Design review of the part built by this model. Coordinates are the model's own, in mm. Face numbers are marked on the shaded views. Give positions to 0.01 mm unless a question says otherwise; leave off trailing zeros. Write each loop counter-clockwise with the first axis right and the second up, starting at its lowest first coordinate (ties: lowest second). Pieces come first, ordered by that corner, then holes. Notation, with made-up numbers: M 17,54 L 34,54 A17 ccw 34,68 Z; hole C 20,-36.5 d11. An arc over 180 degrees is marked long. Use a Markdown table: item, result. Add a question column.
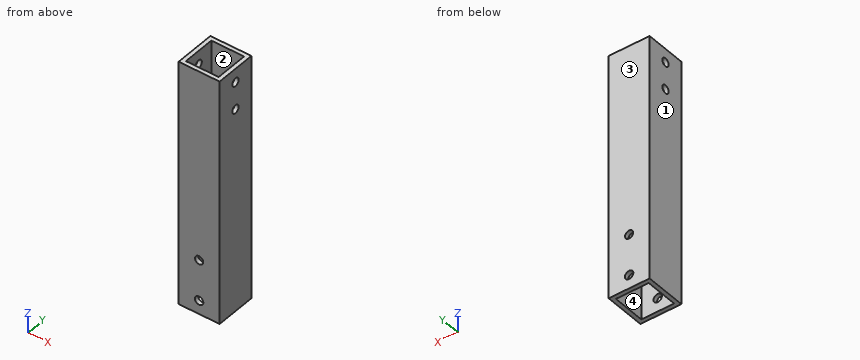
```python
from build123d import *

# Parameters (mm, degrees)
ESQUISSE1_W             = 15
ESQUISSE1_H             = 15
EXTRUSION1_DEPTH        = 90
ESQUISSE2_W             = 12
ESQUISSE2_H             = 12
EXTRUSION2_DEPTH        = 91.622844802
ESQUISSE3_R             = 1.5
ENL_V_MAT_EXTRU_1_DEPTH = 92.549167118
ESQUISSE4_R             = 1.5
ESQUISSE4_R_2           = 1.538778498
ENL_V_MAT_EXTRU_2_DEPTH = 92.549167118


with BuildPart() as part:
    # Esquisse1 → Extrusion1 (new body)
    with BuildSketch(Plane.XY):
        Rectangle(ESQUISSE1_W, ESQUISSE1_H)
    extrude(amount=EXTRUSION1_DEPTH)

    # Esquisse2 → Extrusion2 (cut, through all)
    with BuildSketch(Plane.XY.offset(90)):
        Rectangle(ESQUISSE2_W, ESQUISSE2_H)
    extrude(amount=-EXTRUSION2_DEPTH, mode=Mode.SUBTRACT)

    # Esquisse3 → Enlèv. mat.-Extru.1 (cut, through all)
    with BuildSketch(Plane(origin=(7.5, 0, 0), x_dir=(0, 0, -1), z_dir=(1, 0, 0))):
        with Locations((-85, 0)):
            Circle(ESQUISSE3_R)
        with Locations((-75, 0)):
            Circle(ESQUISSE3_R)
    extrude(amount=-ENL_V_MAT_EXTRU_1_DEPTH, mode=Mode.SUBTRACT)

    # Esquisse4 → Enlèv. mat.-Extru.2 (cut, through all)
    with BuildSketch(Plane(origin=(0, 7.5, 0), x_dir=(1, 0, 0), z_dir=(0, 1, 0))):
        with Locations(Location((0, -20, 0), (0, 0, 270))):
            Circle(ESQUISSE4_R)
        with Locations(Location((0, -5, 0), (0, 0, 270))):
            Circle(ESQUISSE4_R_2)
    extrude(amount=-ENL_V_MAT_EXTRU_2_DEPTH, mode=Mode.SUBTRACT)


solid = part.part
```
(1) Wall thickness on L1, parallel to X at y = 5.5, z = 58.5; L2, parallel to X at y = -6.7, z = 20: over which ranges is each line inside the solid? List them lowest first.
(2) Add section B-B on z = 5. Give the boundary of the cut face in (x, y), then the cut area to 3 significant figures.
(3) The part is to be moulded in two halves that separate along X. For the marked faces 1, 2, 3 and 4, say which applies: released by +X, released by -X, zero draft, split by the parting line, or undercut.
(4) Add section C-C on x = 0. Give the boundary of the cut face in (y, z).
(5) Add section D-D on y = 3.5. Give the boundary of the cut face in (x, z).
(6) For pin 1 (5 mm diameter, centred on x = 0, z = 5, fed in from +Y), flat-tipped, find the tip position at first contact; note if it passes through.
(7) Add section A-A on y = 0. Give the boundary of the cut face in (x, z), then the cut area to 3 significant figures.
From the geometry:
| question | item | result |
|---|---|---|
| 1 | L1 | x = -7.5 to -6, 6 to 7.5 |
| 1 | L2 | x = -7.5 to -1.5, 1.5 to 7.5 |
| 2 | outline | M -7.5,-7.5 L -1.54,-7.5 L -1.54,-6 L -6,-6 L -6,6 L -1.54,6 L -1.54,7.5 L -7.5,7.5 Z; M 1.54,-7.5 L 7.5,-7.5 L 7.5,7.5 L 1.54,7.5 L 1.54,6 L 6,6 L 6,-6 L 1.54,-6 Z |
| 2 | area | 71.8 mm^2 |
| 3 | face 1 | released by -X |
| 3 | face 2 | undercut |
| 3 | face 3 | zero draft |
| 3 | face 4 | undercut |
| 4 | outline | M -7.5,0 L -6,0 L -6,3.46 L -7.5,3.46 Z; M -7.5,6.54 L -6,6.54 L -6,18.5 L -7.5,18.5 Z; M -7.5,21.5 L -6,21.5 L -6,90 L -7.5,90 Z; M 6,0 L 7.5,0 L 7.5,3.46 L 6,3.46 Z; M 6,6.54 L 7.5,6.54 L 7.5,18.5 L 6,18.5 Z; M 6,21.5 L 7.5,21.5 L 7.5,90 L 6,90 Z |
| 5 | outline | M -7.5,0 L -6,0 L -6,90 L -7.5,90 Z; M 6,0 L 7.5,0 L 7.5,90 L 6,90 Z |
| 6 | pin 1 | stops at y = 7.5 |
| 7 | outline | M -7.5,0 L -6,0 L -6,73.5 L -7.5,73.5 Z; M -7.5,76.5 L -6,76.5 L -6,83.5 L -7.5,83.5 Z; M -7.5,86.5 L -6,86.5 L -6,90 L -7.5,90 Z; M 6,0 L 7.5,0 L 7.5,73.5 L 6,73.5 Z; M 6,76.5 L 7.5,76.5 L 7.5,83.5 L 6,83.5 Z; M 6,86.5 L 7.5,86.5 L 7.5,90 L 6,90 Z |
| 7 | area | 252 mm^2 |
